from build123d import *

# Parameters (mm, degrees)
F1_DEPTH = 1.5
F3_DEPTH = 1
F5_DEPTH = 1.5
F6_R     = 1.5
F7_W     = 11
F7_H     = 3.5
F8_DEPTH = 25


with BuildPart() as f1:
    # F0 (on Top) → F1 (new body)
    with BuildSketch(Plane.XY):
        Polygon((6.468732, 38.072392), (-7.768678, 38.072392), (-22.119725, 15.095294), (-20.680386, 6.932392), (19.38044, 6.932392), (20.81978, 15.095294), align=None)
    extrude(amount=F1_DEPTH)

    # F2 (on face) → F3 (join)
    with BuildSketch(Plane(origin=(0, 0, 0), x_dir=(1, 0, 0), z_dir=(0, 0, -1))):
        Polygon((-18.163087, -9.932392), (-18.965392, -14.482494), (-6.105343, -35.072392), (4.805398, -35.072392), (17.665447, -14.482494), (16.863141, -9.932392), align=None)
        Polygon((4.250953, -34.072392), (-5.550899, -34.072392), (-17.913948, -14.278227), (-17.323987, -10.932392), (16.024041, -10.932392), (16.614002, -14.278227), align=None, mode=Mode.SUBTRACT)
    extrude(amount=F3_DEPTH)

    # F4 (on face) → F5 (join)
    with BuildSketch(Plane(origin=(0, 0, 0), x_dir=(1, 0, 0), z_dir=(0, 0, -1))):
        Polygon((16.863141, -6.932392), (16.863141, -9.932392), (16.586395, -19.072392), (23.415447, -19.072392), (22.113141, -6.932392), align=None)
    extrude(amount=-F5_DEPTH)

    # F6
    f6_edges = [f1.edges().sort_by_distance(p)[0] for p in [
        (23.415447, 19.072392, 0.75),
        (18.335762, 19.072392, 0.75),
        (22.113141, 6.932392, 0.75),
        (-20.680386, 6.932392, 0.75),
        (-22.119725, 15.095294, 0.75),
        (-7.768678, 38.072392, 0.75),
        (6.468732, 38.072392, 0.75),
        (4.805398, 35.072392, -0.5),
        (-6.105343, 35.072392, -0.5),
        (-18.965392, 14.482494, -0.5),
        (-18.163087, 9.932392, -0.5),
        (16.863141, 9.932392, -0.5),
        (17.665447, 14.482494, -0.5),
        (-17.323987, 10.932392, -0.5),
        (-17.913948, 14.278227, -0.5),
        (-5.550899, 34.072392, -0.5),
        (4.250953, 34.072392, -0.5),
        (16.024041, 10.932392, -0.5),
        (16.614002, 14.278227, -0.5),
    ]]
    fillet(f6_edges, radius=F6_R)

    # F7 (on face) → F8 (cut)
    with BuildSketch(Plane.XY.offset(1.5)):
        with Locations((-0.649973, 31.422392)):
            Rectangle(F7_W, F7_H)
    extrude(amount=-F8_DEPTH, mode=Mode.SUBTRACT)


solid = f1.part
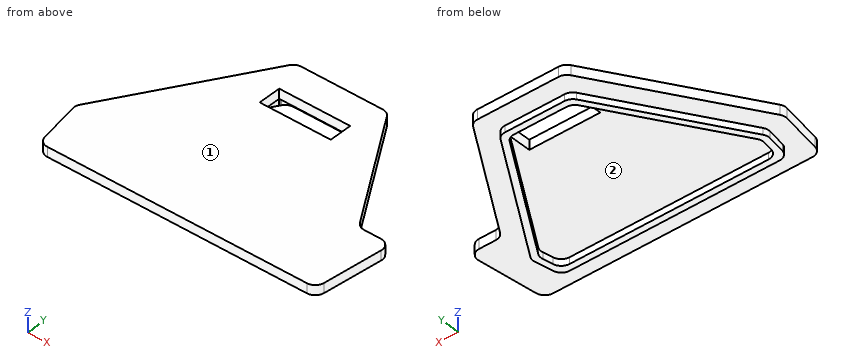
Design review of the part built by this model. Coordinates are the model's own, in mm. Face numbers are marked on the shaded views. Give positions to 0.01 mm unless a question says otherwise; leave off trailing zeros. Loops run counter-clockwise (first coordinate to the right, second up) from the corner with the lowest first, then second, coordinate; pieces in that order, holes last. Notation, with made-up numbers: M 41,56.5 L 55,56.5 A29 cw 55,95.5 Z; hole C 56.25,74.25 d1. An arc over 180 degrees is marked long. One line per question, with ' | ' between items. Start each with the question number.
1. Add section D-D (x = -11.5). Write out the cut boundary in (y, z), plus the area to 3 significant figures.
2. Insertion check: P1, Ø1.5, axis at y = 29.5, z = -0.5, coming from the +X side; P2, Ø3, axis at x = -12.5, y = 16, coming from the -Z side; P3, Ø0.8, axis at y = 32, z = 0, coming from the -X side. Each pin has a flat end and moves straight along its axis. Give the tip position at first contact, or say it passes through.
3. Add section A-A (x = -1.5). Write out the cut boundary in (y, z).
4. The part is to be moulded in two halves that separate along Y. For the marked faces 1 and 2, say which applies: released by +Y, released by -Y, zero draft, split by the parting line, or undercut.
5. Add section C-C (y = 29). Write out the cut boundary in (x, z).
6. To check wall thickness, follow L1, parallel to Z at x = 3, y = 20; L2, parallel to X at y = 17, z = -0.65; L3, parallel to Y at x = -16.5, z = -0.1. State the ranges of each line that lie inside material, in increasing order.
Worked out:
1) outline: M 6.93,0 L 9.93,0 L 9.93,-1 L 10.93,-1 L 10.93,0 L 24.55,0 L 24.55,-1 L 26.44,-1 L 26.44,0 L 32.1,0 L 32.1,1.5 L 6.93,1.5 Z | area: 40.6 mm²
2) P1: stops at x = 12.17 | P2: stops at z = 0 | P3: stops at x = -11.81
3) outline: M 6.93,0 L 9.93,0 L 9.93,-1 L 10.93,-1 L 10.93,0 L 29.67,0 L 29.67,1.5 L 6.93,1.5 Z; M 33.17,0 L 34.07,0 L 34.07,-1 L 35.07,-1 L 35.07,0 L 38.07,0 L 38.07,1.5 L 33.17,1.5 Z
4) face 1: zero draft | face 2: undercut
5) outline: M -13.44,0 L -9.9,0 L -9.9,-1 L -8.72,-1 L -8.72,0 L 7.42,0 L 7.42,-1 L 8.6,-1 L 8.6,0 L 12.14,0 L 12.14,1.5 L -13.44,1.5 Z
6) L1: z = 0 to 1.5 | L2: x = -17.39 to -16.21, 14.91 to 16.09 | L3: y = 9.93 to 11, 16.54 to 18.43
